Can you work these out from the drawing? Everything is in mm from the part's minimum corner. A direction names the side the tool comes from. Round coordinates to 2 decimals unless told otherwise and drop trailing zeros. Write each loop counter-clockwise with the first axis right and the second up, starting at its lowest first coordinate (ties: lowest second). Pieces come first, ordered by that corner, then holes. Notation, with made-up numbers: (38.25, 87.5) -> (92.25, 87.5) arc R23 ccw to (92.25, 123.5) -> close; hole circle Ø8 at (70.25, 2.25). An arc over 180 degrees is marked (long way). Answer as CSV lines item,"result". Start each with the question number.
Q1. If we mould it in two halves opening along Y, with no side actions, what happens to the marked faces 1, 2 and 3? For each: pulls with the +Y half, pulls with the -Y half, needs draft (parallel to the pull), parting line crosses it, or undercut.
Q2. Imagine slicing it at D-D on x = 10.75. Please give me the cut outline in (y, z) (1 decimal).
Q3. Imagine slicing it at C-C on y = 34. Please give me the cut outline in (x, z) (1 decimal).
Q4. For the marked faces 4, 5, 6, 7 and 8, which set-ups out of +Z, -Z, +X, -X, +Y, -Y let a thin tool reach every point of the face, with its end or its side?
Q5. If I drill on line 1 (Y direction, x = 10.25, z = 3.15) (1 decimal); line 2 (X direction, y = 19.5, z = 1); line 3 (X direction, y = 28.5, z = 3.7) (1 decimal), over which ranges is the centre line in solid material (lowest first)? Write a range as [from, to].
Q6. Imagine slicing it at B-B on x = 13.75. Please give me the cut outline in (y, z) (1 decimal), and give its area (3 significant figures).
Q7. Will these pins go through, and if not, where does the flat tip stop? pin 1 Ø1.6 at (x, z) = (2, 2.5) entering from -Y; pin 2 Ø2 at (y, z) = (32, 1.5) entering from -X; pin 3 Ø1 at (x, z) = (7, 2) entering from -Y; pin 4 Ø1.3 at (y, z) = (32, 2.5) entering from +X (3 decimals).
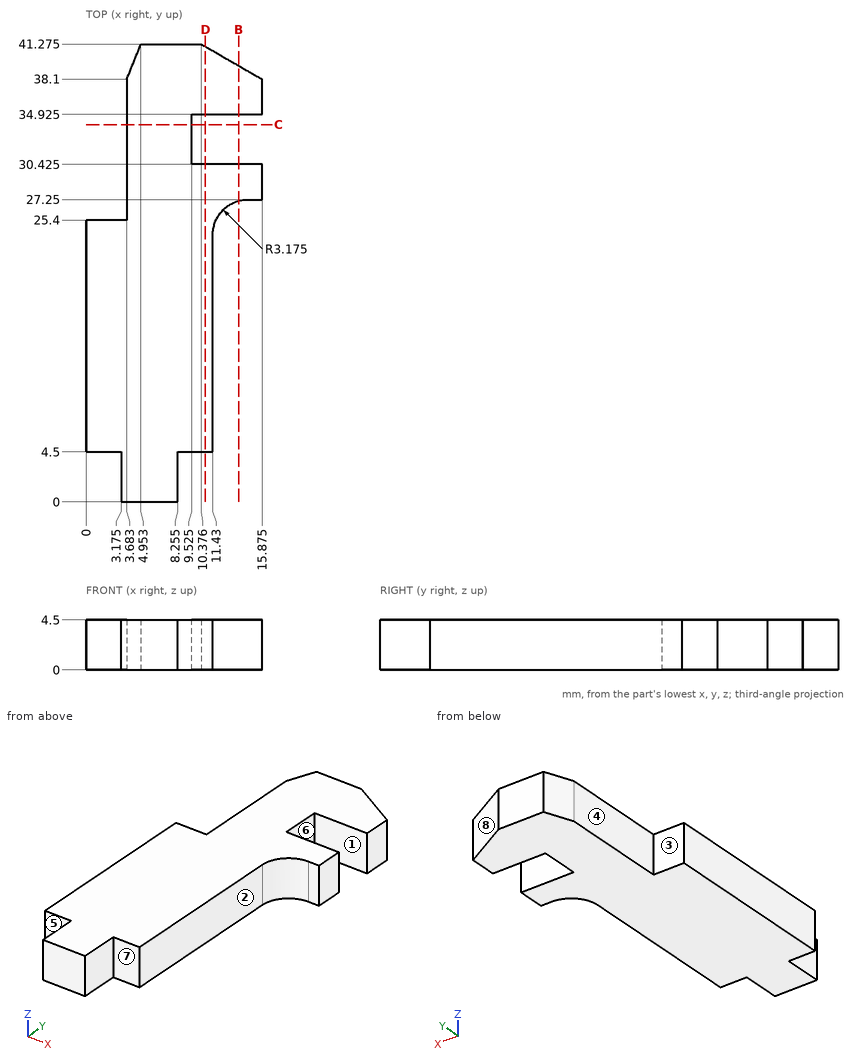
Checks:
1,face 1,"undercut"
1,face 2,"needs draft"
1,face 3,"pulls with the +Y half"
2,outline,"(4.5, 0) -> (30.4, 0) -> (30.4, 4.5) -> (4.5, 4.5) -> close; (34.9, 0) -> (41.1, 0) -> (41.1, 4.5) -> (34.9, 4.5) -> close"
3,outline,"(3.7, 0) -> (9.5, 0) -> (9.5, 4.5) -> (3.7, 4.5) -> close"
4,face 4,"+Z, -Z, -X, +Y"
4,face 5,"+Z, -Z, -X, -Y"
4,face 6,"+Z, -Z, +X"
4,face 7,"+Z, -Z, +X, -Y"
4,face 8,"+Z, -Z, +X, +Y"
5,line 1,"[4.5, 30.4], [34.9, 41.3]"
5,line 2,"[0, 11.43]"
5,line 3,"[3.7, 15.9]"
6,outline,"(27.1, 0) -> (30.4, 0) -> (30.4, 4.5) -> (27.1, 4.5) -> close; (34.9, 0) -> (39.3, 0) -> (39.3, 4.5) -> (34.9, 4.5) -> close"
6,area,"34.6 mm^2"
7,pin 1,"y = 4.5"
7,pin 2,"x = 3.68"
7,pin 3,"y = 0"
7,pin 4,"x = 9.525"
